Check sheet for the modelled part. Datum: model origin and axes. Units: mm. Round coordinates to 2 decimals unless told otherwise and drop trailing zeros. Write each loop counter-clockwise with the first axis right and the second up, starting at its lowest first coordinate (ties: lowest second). Pieces come first, ordered by that corner, then holes. Notation, with made-up numbers: (88.5, 85.5) -> (145.5, 85.5) arc R14 cw to (145.5, 96.5) -> close; hole circle Ø7 at (51, 86.25). An arc over 180 degrees is marked (long way). Write item = value, one per line.
from build123d import *

# Parameters (mm, degrees)
SKETCH_W    = 46
SKETCH_H    = 36
PAD_DEPTH   = 5
FILLET_R    = 5
FILLET001_R = 5
FILLET002_R = 4


with BuildPart() as part:
    # Sketch → Pad (new body)
    with BuildSketch(Plane.XY):
        Rectangle(SKETCH_W, SKETCH_H)
    extrude(amount=PAD_DEPTH)

    # Fillet
    fillet_edges = [part.edges().sort_by_distance(p)[0] for p in [
        (23, -18, 2.5),
        (23, 18, 2.5),
        (-23, -18, 2.5),
    ]]
    fillet(fillet_edges, radius=FILLET_R)

    # Fillet001
    fillet001_edges = [part.edges().sort_by_distance(p)[0] for p in [
        (-23, 18, 2.5),
    ]]
    fillet(fillet001_edges, radius=FILLET001_R)

    # Fillet002
    fillet002_edges = [part.edges().sort_by_distance(p)[0] for p in [
        (-21.535534, -16.535534, 5),
        (21.535534, -16.535534, 5),
        (0, -18, 5),
        (23, 0, 5),
        (21.535534, 16.535534, 5),
        (0, 18, 5),
        (-21.535534, 16.535534, 5),
        (-23, 0, 5),
    ]]
    fillet(fillet002_edges, radius=FILLET002_R)


solid = part.part
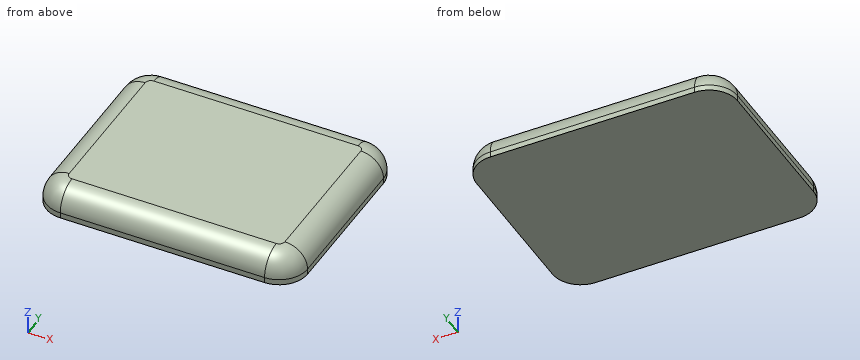
(1) Material ranges on L1, parallel to X at y = 3, z = 1.2 (3 decimals); L2, parallel to X at y = -4.5, z = 2; L3, parallel to Y at x = -11, z = 2.1, recorded low to high. Write a range as [from, to].
Worked answers:
L1 = [-22.995, 22.995]
L2 = [-22.87, 22.87]
L3 = [-17.85, 17.85]
(2) Sectioned sample at A-A on x = 17. Enter the section's corners in (y, z).
Worked answers:
outline = (-18, 0) -> (18, 0) -> (18, 1) arc R4 ccw to (14, 5) -> (-14, 5) arc R4 ccw to (-18, 1) -> close
(3) Sectioned sample at B-B on y = 6. Enter the section's corners in (x, z), then the cut area to 3 significant figures.
Worked answers:
outline = (-23, 0) -> (23, 0) -> (23, 1) arc R4 ccw to (19, 5) -> (-19, 5) arc R4 ccw to (-23, 1) -> close
area = 223 mm²
(4) Go/stop test with flat-tipped pins: P1, Ø12, axis at x = 15, y = -1.5, coming from the -Z side; P2, Ø1, axis at x = 11, z = 2.5, coming from the -Y side; P3, Ø1, axis at y = -11.5, z = 2.5, coming from the -X side. Record where each tip stops, or that it passes through.
Worked answers:
P1 = 0
P2 = -17.87
P3 = -22.87
